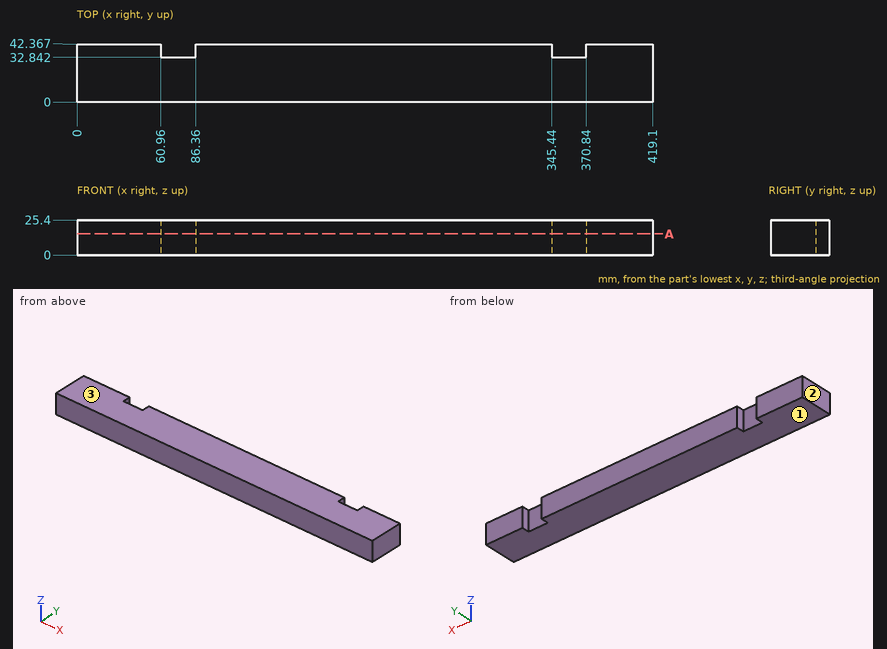
Job drawing, mm, ordinate dimensions from the low corner. One solid piece. Give positions to 0.01 mm unless a question says otherwise; leave off trailing zeros. Order: outer loops, then holes, each group sorted by start corner. A loop starts at its lowest first (then second) coordinate and runs counter-clockwise, first axis right, second up. Notation, with made-up numbers: M -24,76.5 L -14,76.5 A19 ccw -14,98.5 Z; hole C -15.75,-20.75 d8. An arc over 180 degrees is marked long. Put each result on its own line as item: value. Start each with the question number.
(1) Drill centre lines: L1, parallel to X at y = 37, z = 17.5; L2, parallel to Y at x = 358.5, z = 18.75. Where is each one in solid material? Low to high. Write a range as [from, to].
(2) Band-saw the part on A-A on z = 15.5. Give the cut face in (x, y).
(3) Pull direction Z, two halves, no side cores. Call the marked faces 1, 2 and 3: released by +Z, released by -Z, zero draft, split by the parting line, or undercut.
Results below:
1. L1: x = [0, 60.96], [86.36, 345.44], [370.84, 419.1]
1. L2: y = [0, 32.84]
2. outline: M 0,0 L 419.1,0 L 419.1,42.37 L 370.84,42.37 L 370.84,32.84 L 345.44,32.84 L 345.44,42.37 L 86.36,42.37 L 86.36,32.84 L 60.96,32.84 L 60.96,42.37 L 0,42.37 Z
3. face 1: released by -Z
3. face 2: zero draft
3. face 3: released by +Z
